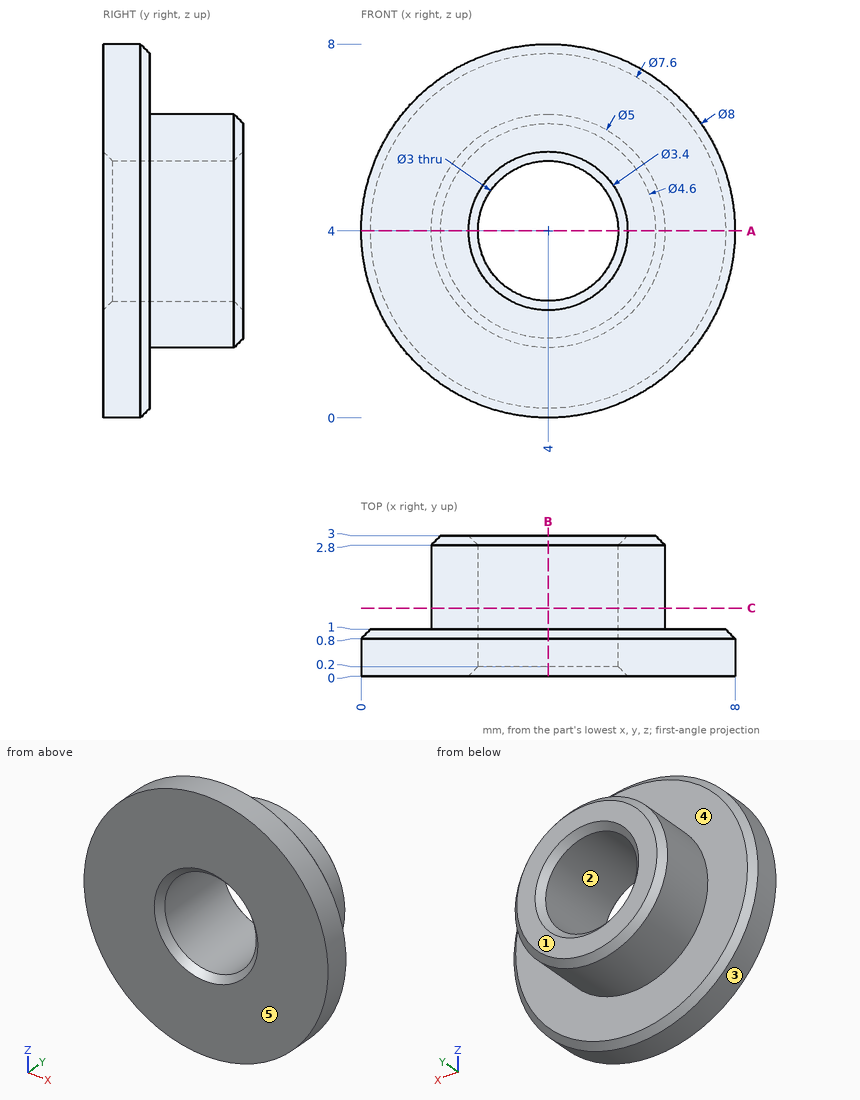
For this review, use the dimensioned drawing (mm, ordinates from the lowest corner) and the shaded views. A direction names the side the tool comes from. Coordinates: 2 decimals unless noted, no trailing zeros. Order: outer loops, then holes, each group sorted by start corner. A loop starts at its lowest first (then second) coordinate and runs counter-clockwise, first axis right, second up. Notation, with made-up numbers: (23, 56.5) - (62, 56.5) arc R8 ccw to (62, 60.5) - close; hole circle Ø10 at (53.25, 58.25). An arc over 180 degrees is marked (long way). Answer as a JSON object with one key per item and string values. Group by question number.
1. We need section B-B on x = 4. State the section outline as (y, z) points, then the cut area to 3 significant figures.
2. For the marked faces 4 and 5, list the 3-axis set-ups (+Z, -Z, +X, -X, +Y, -Y) from which the entire face can be reached by the end or side of a thin tool; tool diameter is ignored.
3. We need section A-A on z = 4. State the section outline as (x, y) points, then the cut area to 3 significant figures.
4. Clearance check with flat-ended pins moving along their axes: P1, Ø2.5, axis at x = 4, z = 4, coming from the +Y side (3 decimals); P2, Ø1, axis at y = 0.5, z = 6, coming from the +X side. State where each tip first meets the part, or that it passes through.
5. We need section C-C on y = 1.45. State the section outline as (x, z) points, then the cut area to 3 significant figures.
6. For probe 1 along X at (y, z) = (1.3, 4); probe 2 along Y at (x, z) = (4, 6.75); probe 3 along X at (y, z) = (1.1, 2.75), list the stretches that pass through material, from the lowest coordinate up.
7. The part is to be moulded in two halves that separate along X. For the marked faces 1, 2 and 3, say which applies: pulls with the +X half, pulls with the -X half, needs draft (parallel to the pull), parting line crosses it, or undercut.
Final values:
{
 "1": {"outline": "(0, 0) - (0.8, 0) - (1, 0.2) - (1, 1.5) - (2.8, 1.5) - (3, 1.7) - (3, 2.3) - (2.8, 2.5) - (0.2, 2.5) - (0, 2.3) - close; (0, 5.7) - (0.2, 5.5) - (2.8, 5.5) - (3, 5.7) - (3, 6.3) - (2.8, 6.5) - (1, 6.5) - (1, 7.8) - (0.8, 8) - (0, 8) - close", "area": "8.84 mm²"},
 "2": {"face 4": "+Y", "face 5": "+Z, -Z, +X, -X, -Y"},
 "3": {"outline": "(0, 0) - (2.3, 0) - (2.5, 0.2) - (2.5, 2.8) - (2.3, 3) - (1.7, 3) - (1.5, 2.8) - (1.5, 1) - (0.2, 1) - (0, 0.8) - close; (5.5, 0.2) - (5.7, 0) - (8, 0) - (8, 0.8) - (7.8, 1) - (6.5, 1) - (6.5, 2.8) - (6.3, 3) - (5.7, 3) - (5.5, 2.8) - close", "area": "8.84 mm²"},
 "4": {"P1": "through", "P2": "x = 7.71"},
 "5": {"outline": "circle Ø5 at (4, 4); hole circle Ø3 at (4, 4)", "area": "12.6 mm²"},
 "6": {"probe 1": "1.5 to 2.5, 5.5 to 6.5", "probe 2": "0 to 1", "probe 3": "1.83 to 3.17, 4.83 to 6.17"},
 "7": {"face 1": "needs draft", "face 2": "undercut", "face 3": "parting line crosses it"}
}
